Work out the finished part from the listing and answer in its coordinate system (mm). Round coordinates to 2 decimals unless told otherwise and drop trailing zeros. Loops run counter-clockwise (first coordinate to the right, second up) from the corner with the lowest first, then second, coordinate; pieces in that order, holes last. Notation, with made-up numbers: (83, 29.5) - (135, 29.5) arc R34 ccw to (135, 67.5) - close; hole circle Ø3 at (-30.5, 53). An arc over 180 degrees is marked (long way). Return JSON: item names as keys, results as strings.
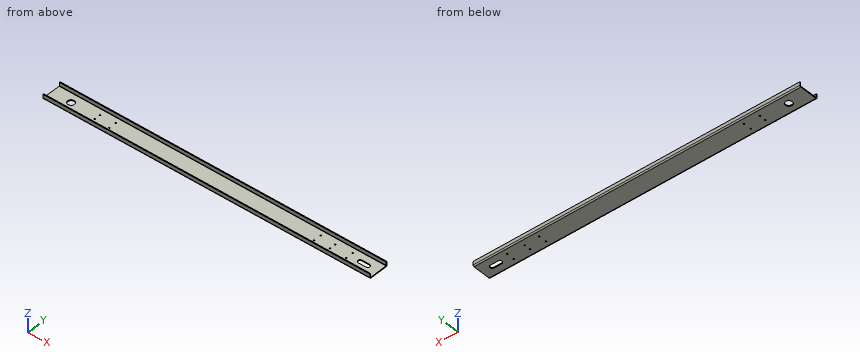
from build123d import *

# Parameters (mm, degrees)
TABAN_FLAN_1_DEPTH    = 535
KES_EKSTR_ZYON1_DEPTH = 10
M5_DI_LI_DELIK1_D     = 4.2
M5_DI_LI_DELIK2_D     = 4.2
M5_DI_LI_DELIK3_D     = 4.2
IZIM13_R              = 11
KES_EKSTR_ZYON2_DEPTH = 10


# Sheet-metal steps are written as plain solids
with BuildPart() as part:
    # Çizim1 → Taban-Flanş1 (new, symmetric)
    with BuildSketch(Plane(origin=(0, 0, 0), x_dir=(0, 0, -1), z_dir=(1, 0, 0))):
        with BuildLine():
            Line((-15, -32.5), (-3.7366, -32.5))
            ThreePointArc((-3.7366, -32.5), (-1.094424801, -31.405575199), (0, -28.7634))
            Line((0, -28.7634), (0, 28.7634))
            ThreePointArc((0, 28.7634), (-1.094424801, 31.405575199), (-3.7366, 32.5))
            Line((-3.7366, 32.5), (-15, 32.5))
            Line((-15, 32.5), (-15, 29.5))
            Line((-15, 29.5), (-3.7366, 29.5))
            ThreePointArc((-3.7366, 29.5), (-3.215745145, 29.284254855), (-3, 28.7634))
            Line((-3, 28.7634), (-3, -28.7634))
            ThreePointArc((-3, -28.7634), (-3.215745145, -29.284254855), (-3.7366, -29.5))
            Line((-3.7366, -29.5), (-15, -29.5))
            Line((-15, -29.5), (-15, -32.5))
        make_face()
    extrude(amount=TABAN_FLAN_1_DEPTH, both=True)

    # Çizim6 → Kes-Ekstrüzyon1 (cut)
    with BuildSketch(Plane(origin=(0, 0, 0), x_dir=(-1, 0, 0), z_dir=(0, 0, -1))):
        with BuildLine():
            Line((-500, 7), (-475, 7))
            ThreePointArc((-475, 7), (-468, 0), (-475, -7))
            Line((-475, -7), (-500, -7))
            ThreePointArc((-500, -7), (-507, 0), (-500, 7))
        make_face()
    extrude(amount=-KES_EKSTR_ZYON1_DEPTH, mode=Mode.SUBTRACT)

    # M5 Dişli Delik1 (through all)
    with Locations(Plane(origin=(440, 12.5, 0), x_dir=(-1, 0, 0), z_dir=(0, 0, -1))):
        with Locations((0, 0), (0, -25)):
            Hole(M5_DI_LI_DELIK1_D / 2)

    # M5 Dişli Delik2 (through all)
    with Locations(Plane(origin=(385, 10, 0), x_dir=(-1, 0, 0), z_dir=(0, 0, -1))):
        with Locations((0, 0), (0, -20)):
            m5_di_li_delik2 = Hole(M5_DI_LI_DELIK2_D / 2)

    # M5 Dişli Delik3 (through all)
    with Locations(Plane(origin=(335, 12.5, 0), x_dir=(-1, 0, 0), z_dir=(0, 0, -1))):
        with Locations((0, 0), (0, -25)):
            m5_di_li_delik3 = Hole(M5_DI_LI_DELIK3_D / 2)

    # Aynalama1: M5 Dişli Delik2, M5 Dişli Delik3 across plane
    add(m5_di_li_delik2.mirror(Plane(origin=(0, 0, 0), x_dir=(0, 0, 1), z_dir=(1, 0, 0))), mode=Mode.SUBTRACT)
    add(m5_di_li_delik3.mirror(Plane(origin=(0, 0, 0), x_dir=(0, 0, 1), z_dir=(1, 0, 0))), mode=Mode.SUBTRACT)

    # Çizim13 → Kes-Ekstrüzyon2 (cut)
    with BuildSketch(Plane(origin=(0, 0, 0), x_dir=(-1, 0, 0), z_dir=(0, 0, -1))):
        with Locations((471, 0)):
            Circle(IZIM13_R)
    extrude(amount=-KES_EKSTR_ZYON2_DEPTH, mode=Mode.SUBTRACT)


solid = part.part
1) Section B-B (z = 8.5) is taken. Give the vertices of the cut face in (x, y), and give its area (3 significant figures).
Verdict:
{"outline": "(-535, -32.5) - (535, -32.5) - (535, -29.5) - (-535, -29.5) - close; (-535, 29.5) - (535, 29.5) - (535, 32.5) - (-535, 32.5) - close", "area": "6,420 mm2"}
2) Section C-C (x = -123) is taken. Give the vertices of the cut face in (y, z), and give its area (3 significant figures).
Verdict:
{"outline": "(-32.5, 3.74) arc R3.74 ccw to (-28.76, 0) - (28.76, 0) arc R3.74 ccw to (32.5, 3.74) - (32.5, 15) - (29.5, 15) - (29.5, 3.74) arc R0.74 cw to (28.76, 3) - (-28.76, 3) arc R0.74 cw to (-29.5, 3.74) - (-29.5, 15) - (-32.5, 15) - close", "area": "261 mm2"}
3) Find the intervals of material crossed by L1, parallel to Y at x = -76, z = 14.25; L2, parallel to Y at x = -285, z = 3.25; L3, parallel to Y at x = 440, z = 2.1, in increasing order.
Verdict:
{"L1": "y = -32.5 to -29.5, 29.5 to 32.5", "L2": "y = -32.47 to -29.32, 29.32 to 32.47", "L3": "y = -32.12 to -14.6, -10.4 to 10.4, 14.6 to 32.12"}
4) Flat-ended cylindrical pins translate along their axes: pin 1 (4 mm diameter, centred on x = -133.5, y = -10, fed in from +Z); pin 2 (0.9 mm diameter, centred on x = 489, z = 1.5, fed in from -Y); pin 3 (3.5 mm diameter, centred on x = 491.5, z = 1, fed in from +Y). Find the tip coordinate at first contact, or state that the pin passes through.
Verdict:
{"pin 1": "stops at z = 3", "pin 2": "stops at y = -32.05", "pin 3": "stops at y = 32.37"}
5) Section A-A (x = -471) is taken. Give the vertices of the cut face in (y, z).
Verdict:
{"outline": "(-32.5, 3.74) arc R3.74 ccw to (-28.76, 0) - (-11, 0) - (-11, 3) - (-28.76, 3) arc R0.74 cw to (-29.5, 3.74) - (-29.5, 15) - (-32.5, 15) - close; (11, 0) - (28.76, 0) arc R3.74 ccw to (32.5, 3.74) - (32.5, 15) - (29.5, 15) - (29.5, 3.74) arc R0.74 cw to (28.76, 3) - (11, 3) - close"}
